Can you work these out from the drawing? Everything is in mm from the part's minimum corner. A direction names the side the tool comes from. Round coordinates to 2 decimals unless told otherwise and drop trailing zeros. Order: outer loops, then holes, each group sorted by start corner. A loop starts at its lowest first (then second) coordinate and runs counter-clockwise, first axis right, second up. Notation, with made-up numbers: (-18, 84) -> (6, 84) arc R24 cw to (6, 112) -> close; hole circle Ø5 at (84.5, 53.25). An arc over 180 degrees is marked (long way). Use a Markdown table: item, result. Add a question column.
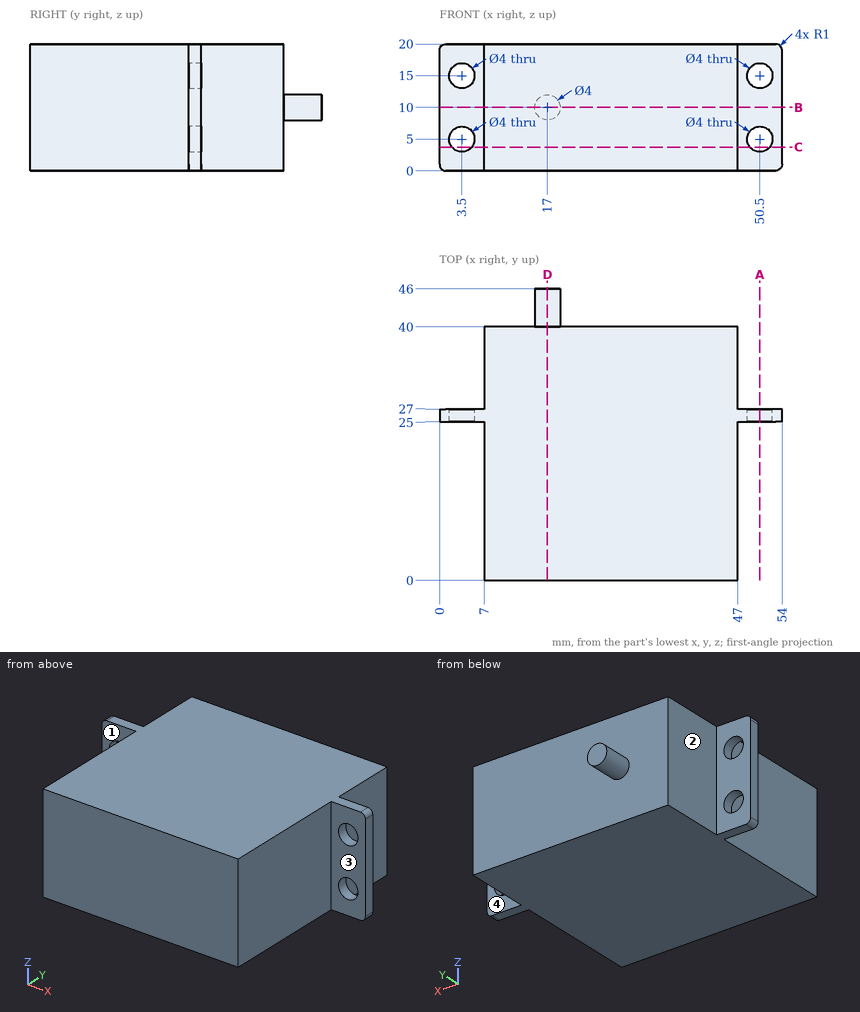
(1) I'm going to push flat-ended pins straight in: P1, Ø7.5, axis at x = 50.5, z = 14, coming from the +Y side; P2, Ø6.5, axis at y = 33, z = 8, coming from the -X side; P3, Ø5, axis at y = 22, z = 8.5, coming from the +X side. Where does each tip first touch, or does it pass through?
(2) On a 3-axis mill with a long thin cutter (end or side, diameter ignored), from which of +Z, -Z, +X, -X, +Y, -Y can I reach the whole of each face in a straight line? I mean the marked faces 1, 2, 3 and 4. Say none if no direction works.
(3) I want a section at B-B on z = 10. List the corners of the cut face in (x, y) for me.
(4) I want a section at A-A on x = 50.5. List the corners of the cut face in (y, z) for me, and give its area (3 significant figures).
(5) I want a section at D-D on x = 17. List the corners of the cut face in (y, z) for me.
(6) Please list where these lines run through material, in increasing order: probe 1 along X at (y, z) = (25.6, 5); probe 2 along Y at (x, z) = (29, 4.75); probe 3 along Y at (x, z) = (49, 1.5). Write a range as from..to.
(7) I want a section at C-C on z = 3.75. List the corners of the cut face in (x, y) for me.
Output:
| question | item | result |
|---|---|---|
| 1 | P1 | y = 40 |
| 1 | P2 | x = 7 |
| 1 | P3 | x = 47 |
| 2 | face 1 | +Z, -Z, -X, -Y |
| 2 | face 2 | +Z, -Z, -X, +Y |
| 2 | face 3 | +Z, -Z, +X, -Y |
| 2 | face 4 | +Z, -Z, +X, +Y |
| 3 | outline | (0, 25) -> (7, 25) -> (7, 0) -> (47, 0) -> (47, 25) -> (54, 25) -> (54, 27) -> (47, 27) -> (47, 40) -> (19, 40) -> (19, 46) -> (15, 46) -> (15, 40) -> (7, 40) -> (7, 27) -> (0, 27) -> close |
| 4 | outline | (25, 0) -> (27, 0) -> (27, 3) -> (25, 3) -> close; (25, 7) -> (27, 7) -> (27, 13) -> (25, 13) -> close; (25, 17) -> (27, 17) -> (27, 20) -> (25, 20) -> close |
| 4 | area | 24.0 mm² |
| 5 | outline | (0, 0) -> (40, 0) -> (40, 8) -> (46, 8) -> (46, 12) -> (40, 12) -> (40, 20) -> (0, 20) -> close |
| 6 | probe 1 | 0..1.5, 5.5..48.5, 52.5..54 |
| 6 | probe 2 | 0..40 |
| 6 | probe 3 | 25..27 |
| 7 | outline | (0, 25) -> (1.94, 25) -> (1.94, 27) -> (0, 27) -> close; (5.06, 25) -> (7, 25) -> (7, 0) -> (47, 0) -> (47, 25) -> (48.94, 25) -> (48.94, 27) -> (47, 27) -> (47, 40) -> (7, 40) -> (7, 27) -> (5.06, 27) -> close; (52.06, 25) -> (54, 25) -> (54, 27) -> (52.06, 27) -> close |
